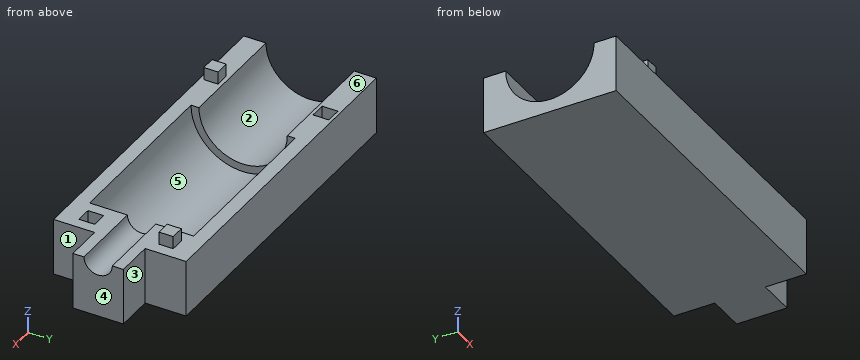
from build123d import *

# Parameters (mm, degrees)
F0_W      = 80
F0_H      = 42
F1_DEPTH  = 22
F3_DEPTH  = 80
F4_DEPTH  = 2
F6_DEPTH  = 22
F7_DEPTH  = 28
F8_DEPTH  = 15
F9_DEPTH  = 2
F10_DEPTH = 10
F11_W     = 5
F11_H     = 5
F12_DEPTH = 4
F11_W_2   = 4.5
F11_H_2   = 4.5
F13_DEPTH = 4
F14_DEPTH = 12
F15_DEPTH = 4
F16_W     = 13
F16_H     = 18
F17_DEPTH = 12


# Not quite as in the source:
# - a feature names something its author has since deleted; it is built from what else it names


with BuildPart() as f1:
    # F0 (on Top) → F1 (new body)
    with BuildSketch(Plane.XY):
        Rectangle(F0_W, F0_H)
    extrude(amount=F1_DEPTH)

    # F2 (on face) → F3 (cut)
    with BuildSketch(Plane.YZ.offset(40)):
        with BuildLine():
            ThreePointArc((-16.5, 22), (0, 5.5), (16.5, 22))
            Line((16.5, 22), (14, 22))
            ThreePointArc((14, 22), (0, 8), (-14, 22))
            Line((-14, 22), (-16.5, 22))
        make_face()
        with BuildLine():
            ThreePointArc((-14, 22), (0, 8), (14, 22))
            Line((14, 22), (4.5, 22))
            ThreePointArc((4.5, 22), (0, 17.5), (-4.5, 22))
            Line((-4.5, 22), (-14, 22))
        make_face()
        with BuildLine():
            ThreePointArc((-4.5, 22), (0, 17.5), (4.5, 22))
            Line((4.5, 22), (-4.5, 22))
        make_face()
    extrude(amount=-F3_DEPTH, mode=Mode.SUBTRACT)

    # F2 (on face) → F4 (join)
    with BuildSketch(Plane.YZ.offset(40)):
        with BuildLine():
            ThreePointArc((-16.5, 22), (0, 5.5), (16.5, 22))
            Line((16.5, 22), (14, 22))
            ThreePointArc((14, 22), (0, 8), (-14, 22))
            Line((-14, 22), (-16.5, 22))
        make_face()
    extrude(amount=-F4_DEPTH)



with BuildPart() as f6:
    # F5 (on face) → F6 (new body)
    with BuildSketch(Plane(origin=(-40, 0, 0), x_dir=(0, -1, 0), z_dir=(-1, 0, 0))):
        with BuildLine():
            Line((-14, 22), (14, 22))
            ThreePointArc((14, 22), (0, 36), (-14, 22))
        make_face()
    extrude(amount=-F6_DEPTH)


with BuildPart() as f1_1:
    add(f1.part)

    add(f6.part)  # F6#2 merges F6
    # F5 (on face) → F6, piece 2 (join)
    with BuildSketch(Plane(origin=(-40, 0, 0), x_dir=(0, -1, 0), z_dir=(-1, 0, 0))):
        with BuildLine():
            Line((16.5, 22), (14, 22))
            ThreePointArc((14, 22), (0, 8), (-14, 22))
            Line((-14, 22), (-16.5, 22))
            ThreePointArc((-16.5, 22), (0, 5.5), (16.5, 22))
        make_face()
        with BuildLine():
            Line((21, 22), (16.5, 22))
            ThreePointArc((16.5, 22), (0, 5.5), (-16.5, 22))
            Line((-16.5, 22), (-21, 22))
            Line((-21, 22), (-21, 0))
            Line((-21, 0), (21, 0))
            Line((21, 0), (21, 22))
        make_face()
    extrude(amount=-F6_DEPTH)

    # F5 (on face) → F7 (cut)
    with BuildSketch(Plane(origin=(-40, 0, 0), x_dir=(0, -1, 0), z_dir=(-1, 0, 0))):
        with BuildLine():
            Line((-14, 22), (14, 22))
            ThreePointArc((14, 22), (0, 36), (-14, 22))
        make_face()
    extrude(amount=-F7_DEPTH, mode=Mode.SUBTRACT)

    # F8 (add): a face of the model
    f8_faces = [f1_1.faces().sort_by_distance(p)[0] for p in [
        (-40, 0, 0.4741307836),
    ]]
    extrude(f8_faces, amount=F8_DEPTH)

    # F2 (on face) → F9 (join)
    with BuildSketch(Plane.YZ.offset(40)):
        with BuildLine():
            ThreePointArc((-14, 22), (0, 8), (14, 22))
            Line((14, 22), (4.5, 22))
            ThreePointArc((4.5, 22), (0, 17.5), (-4.5, 22))
            Line((-4.5, 22), (-14, 22))
        make_face()
    extrude(amount=-F9_DEPTH)

    # F10 (add): a face of the model
    f10_faces = [f1_1.faces().sort_by_distance(p)[0] for p in [
        (40, 0, 10.6759160757),
    ]]
    extrude(f10_faces, amount=F10_DEPTH)

    # F11 (on face) → F12 (cut)
    with BuildSketch(Plane.XY.offset(22)):
        with Locations((-33, 17.5)):
            Rectangle(F11_W, F11_H)
        with Locations((44, -12.5)):
            Rectangle(F11_W, F11_H)
    extrude(amount=-F12_DEPTH, mode=Mode.SUBTRACT)

    # F11 (on face) → F13 (join)
    with BuildSketch(Plane.XY.offset(22)):
        with Locations((-33, -17.5)):
            Rectangle(F11_W_2, F11_H_2)
        with Locations((44, 12.5)):
            Rectangle(F11_W_2, F11_H_2)
    extrude(amount=F13_DEPTH)

    # F14 (add): a face of the model
    f14_faces = [f1_1.faces().sort_by_distance(p)[0] for p in [
        (50, 0, 10.6759160757),
    ]]
    extrude(f14_faces, amount=F14_DEPTH)

    # F15 (cut): a face of the model
    f15_faces = [f1_1.faces().sort_by_distance(p)[0] for p in [
        (3.5, 0, 0),
    ]]
    extrude(f15_faces, amount=-F15_DEPTH, mode=Mode.SUBTRACT)

    # F16 (on face) → F17 (cut)
    with BuildSketch(Plane.YZ.offset(62)):
        with Locations((-14.5, 13)):
            Rectangle(F16_W, F16_H)
        with Locations((14.5, 13)):
            Rectangle(F16_W, F16_H)
    extrude(amount=-F17_DEPTH, mode=Mode.SUBTRACT)


solid = f1_1.part
For this review, take the finished solid that the model builds, in its own axes (mm). Face numbers are marked on the shaded views. A direction names the side the tool comes from. Round coordinates to 2 decimals unless told otherwise and drop trailing zeros. Loops run counter-clockwise (first coordinate to the right, second up) from the corner with the lowest first, then second, coordinate; pieces in that order, holes last. Notation, with made-up numbers: (81.25, -14) - (98.25, -14) arc R17 cw to (98.25, 3) - close; hole circle Ø7 at (41.25, 51.5). An arc over 180 degrees is marked (long way). Put each result on its own line as item: value. Start each with the question number.
1. Consider section D-D on y = 18. State the section outline as (x, z) points.
2. For probe 1 along Y at (x, z) = (-32.5, 20.5); probe 2 along X at (y, z) = (-12.5, 20.5); probe 3 along X at (y, z) = (6, 21), list the stretches that pass through material, from the lowest coordinate up. Write a range as [from, to].
3. For the marked faces 1, 2 and 3, list the 3-axis set-ups (+Z, -Z, +X, -X, +Y, -Y) from which the entire face can be reached by the end or side of a thin tool; tool diameter is ignored.
4. Consider section C-C on z = 16. State the section outline as (x, y) points, plus the area to 3 significant figures.
5. Consider section A-A on y = 0. State the section outline as (x, z) points.
6. Insertion check: P1, Ø2, axis at x = -34, z = 25, coming from the +Y side; P2, Ø5.5, axis at x = 43, y = -13, coming from the +Z side; P3, Ø3, axis at x = 44.5, z = 24.5, coming from the -Y side; P4, Ø13, axis at x = 54.5, z = 13, coming from the -Y side. Each pin has a flat end and moves straight along its axis. Give the tip position at first contact, or say it passes through.
7. Mouldability with a two-part tool opening along X and no side actions: class the marked faces 4, 5 and 6 as +X half, -X half, draft (parallel to the pull), parting line (faces both ways), or undercut.
8. Consider section B-B on x = 21. State the section outline as (y, z) points.
Result sheet:
1. outline: (-55, 4) - (50, 4) - (50, 22) - (-30.5, 22) - (-30.5, 18) - (-35.5, 18) - (-35.5, 22) - (-55, 22) - close
2. probe 1: [-21, -13.92], [13.92, 15], [20, 21]
2. probe 2: [38, 41.5], [46.5, 50]
2. probe 3: [38, 62]
3. face 1: +Z, -Z, +X, -Y
3. face 2: +Z, -X
3. face 3: +Z, -Z, +X, +Y
4. outline: (-55, -21) - (50, -21) - (50, -8) - (62, -8) - (62, 8) - (50, 8) - (50, 21) - (-55, 21) - (-55, 12.65) - (-18, 12.65) - (-18, 15.37) - (38, 15.37) - (38, -15.37) - (-18, -15.37) - (-18, -12.65) - (-55, -12.65) - close
4. area: 1,940 mm^2
5. outline: (-55, 4) - (62, 4) - (62, 17.5) - (38, 17.5) - (38, 5.5) - (-18, 5.5) - (-18, 8) - (-55, 8) - close
6. P1: y = -15.25
6. P2: z = 22
6. P3: y = 10.25
6. P4: y = -21
7. face 4: +X half
7. face 5: undercut
7. face 6: draft
8. outline: (-21, 4) - (21, 4) - (21, 22) - (16.5, 22) arc R16.5 cw to (-16.5, 22) - (-21, 22) - close
